```python
from build123d import *


with BuildPart() as part:
    # Sketch1 → Revolve1 (revolve)
    with BuildSketch(Plane.XY, mode=Mode.PRIVATE) as revolve1_sk:
        with BuildLine():
            Line((0, 7.285), (0, 5.6))
            ThreePointArc((0, 5.6), (0.175735931, 5.175735931), (0.6, 5))
            Line((0.6, 5), (8.4, 5))
            ThreePointArc((8.4, 5), (8.824264069, 5.175735931), (9, 5.6))
            Line((9, 5.6), (9, 9.15))
            Line((9, 9.15), (7.328427125, 9.15))
            ThreePointArc((7.328427125, 9.15), (5.845030918, 7.468416171), (3.610182603, 7.285))
            Line((3.610182603, 7.285), (0, 7.285))
        make_face()
    revolve(revolve1_sk.sketch.rotate(Axis((9, 0, 0), (-1, 0, 0)), 270), axis=Axis((9, 0, 0), (-1, 0, 0)))


solid = part.part
```
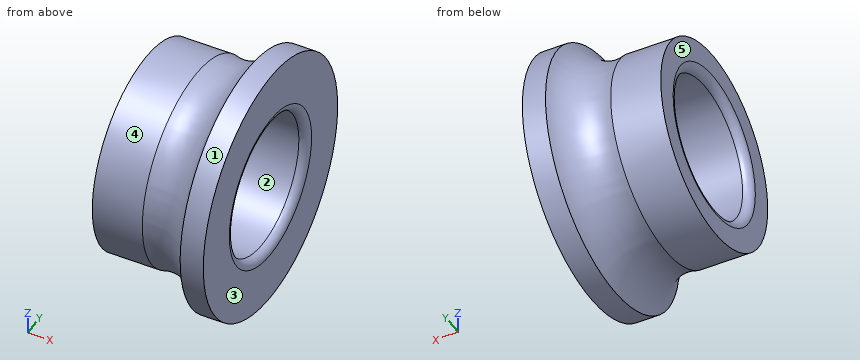
Geometry check sheet. Reference: the model listing, model coordinates, mm. Face numbers are marked on the shaded views. A direction names the side the tool comes from. Coordinates: 2 decimals unless noted, no trailing zeros. Order: outer loops, then holes, each group sorted by start corner. A loop starts at its lowest first (then second) coordinate and runs counter-clockwise, first axis right, second up.
Item 1: Section check D-D (x = 6.75). Enter the section's corners in (y, z), plus the area to 3 significant figures.
Item 2: Scan lines: line 1 along Y through (x, z) = (3.5, 0) (3 decimals); line 2 along Y through (x, z) = (6, 0); line 3 along Z through (x, y) = (2.5, -2.5). Record each from-to range of solid material in increasing order.
Item 3: Depth check by flat-ended pin: pin 1 (1.5 mm diameter, centred on x = 3.5, y = 7, fed in from +Z); pin 2 (2 mm diameter, centred on x = 6, y = 5, fed in from +Z); pin 3 (1 mm diameter, centred on x = 5, y = 5, fed in from -Z); pin 4 (10 mm diameter, centred on y = 1.5, z = -7.5, fed in from -X). Enter the tip coordinate at first touch or a pass-through.
Item 4: Tool access check on the marked faces 4 and 5. Record the directions out of +Z, -Z, +X, -X, +Y, -Y that give a thin tool (end or side, any length) a straight path to the whole face; none if there is none.
Item 5: Section check A-A (y = 0). Enter the section's corners in (x, z) (3 decimals), plus the area to 3 significant figures.
Item 6: Mould release check, pull along Z, two halves, no side actions. Record for the marked faces 1, 2 and 3: released by +Z, released by -Z, zero draft, split by the parting line, or undercut.
Item 7: Section check C-C (x = 1.5). Enter the section's corners in (y, z) (3 decimals).
Check sheet entries:
1. outline: circle Ø16.33 at (0, 0); hole circle Ø10 at (0, 0)
1. area: 131 mm2
2. line 1: y = -7.285 to -5, 5 to 7.285
2. line 2: y = -7.55 to -5, 5 to 7.55
2. line 3: z = -6.84 to -4.33, 4.33 to 6.84
3. pin 1: stops at z = 3.74
3. pin 2: stops at z = 7
3. pin 3: stops at z = -5.63
3. pin 4: stops at x = 0
4. face 4: -X
4. face 5: +Z, -Z, -X, +Y, -Y
5. outline: (0, -7.285) - (3.61, -7.285) arc R3 cw to (7.328, -9.15) - (9, -9.15) - (9, -5.6) arc R0.6 ccw to (8.4, -5) - (0.6, -5) arc R0.6 ccw to (0, -5.6) - close; (0, 5.6) arc R0.6 ccw to (0.6, 5) - (8.4, 5) arc R0.6 ccw to (9, 5.6) - (9, 9.15) - (7.328, 9.15) arc R3 cw to (3.61, 7.285) - (0, 7.285) - close
5. area: 49.2 mm2
6. face 1: split by the parting line
6. face 2: undercut
6. face 3: zero draft
7. outline: circle Ø14.57 at (0, 0); hole circle Ø10 at (0, 0)
